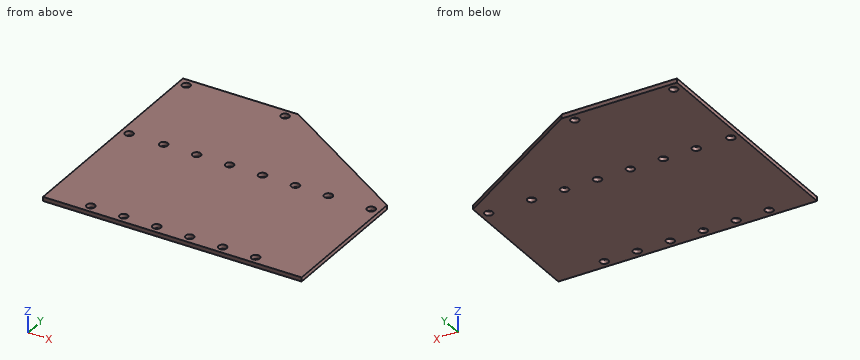
```python
from build123d import *

# Parameters (mm, degrees)
SKETCH1_W           = 199.39
SKETCH1_H           = 177.8
BOSS_EXTRUDE1_DEPTH = 3.175
CUT_EXTRUDE4_DEPTH  = 134.612812447
SKETCH7_R           = 3.175
CUT_EXTRUDE5_DEPTH  = 134.612812447


with BuildPart() as part:
    # Sketch1 → Boss-Extrude1 (new body)
    with BuildSketch(Plane.XY):
        Rectangle(SKETCH1_W, SKETCH1_H)
    extrude(amount=BOSS_EXTRUDE1_DEPTH)

    # Sketch6 → Cut-Extrude4 (cut, through all)
    with BuildSketch(Plane.XY.offset(3.175)):
        Polygon((99.695, 88.9), (99.695, 19.474999912), (-10.795, 88.9), align=None)
    extrude(amount=-CUT_EXTRUDE4_DEPTH, mode=Mode.SUBTRACT)

    # Sketch7 → Cut-Extrude5 (cut, through all)
    with BuildSketch(Plane.XY.offset(3.175)):
        with Locations((-93.345, 82.55)):
            Circle(SKETCH7_R)
        with Locations((-93.345, 9.949999912)):
            Circle(SKETCH7_R)
        with Locations((93.345, 9.949999912)):
            Circle(SKETCH7_R)
        with Locations((-66.675, 9.949999912)):
            Circle(SKETCH7_R)
        with Locations((-41.275, 9.949999912)):
            Circle(SKETCH7_R)
        with Locations((-15.875, 9.949999912)):
            Circle(SKETCH7_R)
        with Locations((9.525, 9.949999912)):
            Circle(SKETCH7_R)
        with Locations((34.925, 9.949999912)):
            Circle(SKETCH7_R)
        with Locations((60.325, 9.949999912)):
            Circle(SKETCH7_R)
        with Locations((-17.145, 82.55)):
            Circle(SKETCH7_R)
        with Locations((-66.675, -82.55)):
            Circle(SKETCH7_R)
        with Locations((-41.275, -82.55)):
            Circle(SKETCH7_R)
        with Locations((-15.875, -82.55)):
            Circle(SKETCH7_R)
        with Locations((9.525, -82.55)):
            Circle(SKETCH7_R)
        with Locations((34.925, -82.55)):
            Circle(SKETCH7_R)
        with Locations((60.325, -82.55)):
            Circle(SKETCH7_R)
    extrude(amount=-CUT_EXTRUDE5_DEPTH, mode=Mode.SUBTRACT)


solid = part.part
```
The listing builds one solid part. Answer for the finished solid, in the listing's coordinates (mm). Round coordinates to 2 decimals unless told otherwise and drop trailing zeros. Loops run counter-clockwise (first coordinate to the right, second up) from the corner with the lowest first, then second, coordinate; pieces in that order, holes last.
Q1. Section A-A, the plane y = -82.55 is taken. Determine the outline of the cut face in (x, z) (3 decimals).
Q2. Section B-B, the plane z = 1.95 is taken. Count the separate pieces of the cut face and the enclosed holes in it, then the cut area to 3 significant figures.
Q3. Given pin 1 Ø7.5 at (x, y) = (-66.675, 9.95) entering from -Z, flat-ended and moving along its own axis, determine where the tip first touches the part or whether it passes through.
Q4. Section C-C, the plane y = 82.55 is taken. Determine the outline of the cut face in (x, z) (3 decimals).
Q5. Find the intervals of material crossed by line 1 (Y direction, x = -44, z = 3); line 2 (Y direction, x = 9.5, z = 1.25); line 3 (X direction, y = 19.5, z = 1) (3 decimals), in increasing order.
Completed:
1. outline: (-99.695, 0) - (-69.85, 0) - (-69.85, 3.175) - (-99.695, 3.175) - close; (-63.5, 0) - (-44.45, 0) - (-44.45, 3.175) - (-63.5, 3.175) - close; (-38.1, 0) - (-19.05, 0) - (-19.05, 3.175) - (-38.1, 3.175) - close; (-12.7, 0) - (6.35, 0) - (6.35, 3.175) - (-12.7, 3.175) - close; (12.7, 0) - (31.75, 0) - (31.75, 3.175) - (12.7, 3.175) - close; (38.1, 0) - (57.15, 0) - (57.15, 3.175) - (38.1, 3.175) - close; (63.5, 0) - (99.695, 0) - (99.695, 3.175) - (63.5, 3.175) - close
2. separate pieces: 1
2. enclosed holes: 16
2. area: 31,100 mm2
3. pin 1: stops at z = 0
4. outline: (-99.695, 0) - (-96.52, 0) - (-96.52, 3.175) - (-99.695, 3.175) - close; (-90.17, 0) - (-20.32, 0) - (-20.32, 3.175) - (-90.17, 3.175) - close; (-13.97, 0) - (-0.689, 0) - (-0.689, 3.175) - (-13.97, 3.175) - close
5. line 1: y = -88.9 to -84.18, -80.92 to 8.32, 11.58 to 88.9
5. line 2: y = -88.9 to -85.72, -79.38 to 6.78, 13.12 to 76.15
5. line 3: x = -99.695 to 99.655
